The listing builds one solid part. Answer for the finished solid, in the listing's coordinates (mm). Face numbers are marked on the shaded views. A direction names the side the tool comes from. Round coordinates to 2 decimals unless told otherwise and drop trailing zeros. Write each loop counter-clockwise with the first axis right and the second up, starting at its lowest first coordinate (ties: lowest second). Pieces come first, ordered by that corner, then holes. Notation, with made-up numbers: (-38, 2.25) - (8, 2.25) arc R16 cw to (8, 18.25) - close; hole circle Ø7 at (55, 77). An arc over 180 degrees is marked (long way). Return JSON: item names as keys, results as strings. Group by question number.
(1) Which of the six approach directions +Z, -Z, +X, -X, +Y, -Y give full straight-line access (tool end or side, diameter ignored) to the marked faces 1 and 2?
(2) Section D-D, the plane z = 16.5 is taken. Write down the section's boundary in (x, y), then the cut area to 3 significant figures.
(3) Section C-C, the plane x = 2.25 is taken. Write down the section's boundary in (y, z), then the cut area to 3 significant figures.
(4) Determine the mould class of the marked faces 3, 4, 5 and 6 for opening direction Z: +Z half, -Z half, draft (parallel to the pull), parting line (faces both ways), or undercut.
(5) Each of these flat-tipped pins is pushed along its axis until it touches: pin 1 (8.5 mm diameter, centred on y = 11, z = 10, fed in from -X); pin 2 (3.5 mm diameter, centred on x = 6, z = 6, fed in from -Y). Where does it stop, or does it pass through?
(6) Find the intervals of material crossed by line 1 along Y through (x, z) = (1.8, 14.75); line 2 along Y through (x, z) = (4.75, 10); line 3 along X through (y, z) = (6.5, 10.5), in increasing order. Write a range as [from, to].
(7) Section A-A, the plane y = 11 is taken. Write down the section's boundary in (x, z), then the cut area to 3 significant figures.
(8) Section B-B, the plane z = 10 is taken. Write down the section's boundary in (x, y).
```python
from build123d import *

# Parameters (mm, degrees)
BOSS_EXTRUDE1_DEPTH = 20
CUT_EXTRUDE1_REACH  = 9
SKETCH2_R           = 2.6
CUT_EXTRUDE2_REACH  = 6
SKETCH3_R           = 1.25


with BuildPart() as part:
    # Sketch1 → Boss-Extrude1 (new body)
    with BuildSketch(Plane.XY):
        Polygon((7, 15), (0, 15), (0, 0), (4, 0), (4, 7), (7, 7), align=None)
    extrude(amount=BOSS_EXTRUDE1_DEPTH)

    # Sketch2 → Cut-Extrude1 (cut, up to next)
    with BuildSketch(Plane(origin=(7, 0, 0), x_dir=(0, 0, -1), z_dir=(1, 0, 0)), mode=Mode.PRIVATE) as cut_extrude1_sk1:
        with Locations((-10, 11)):
            Circle(SKETCH2_R)
    cut_extrude1_tool1 = extrude(cut_extrude1_sk1.sketch, amount=-CUT_EXTRUDE1_REACH, mode=Mode.PRIVATE) & part.part
    add(cut_extrude1_tool1.solids().sort_by_distance((7, 11, 10))[0], mode=Mode.SUBTRACT)

    # Sketch3 → Cut-Extrude2 (cut, up to next)
    with BuildSketch(Plane(origin=(4, 0, 0), x_dir=(0, 0, -1), z_dir=(1, 0, 0)), mode=Mode.PRIVATE) as cut_extrude2_sk1:
        with Locations((-14.75, 3.497875885)):
            Circle(SKETCH3_R)
    cut_extrude2_tool1 = extrude(cut_extrude2_sk1.sketch, amount=-CUT_EXTRUDE2_REACH, mode=Mode.PRIVATE) & part.part
    add(cut_extrude2_tool1.solids().sort_by_distance((4, 3.497876, 14.75))[0], mode=Mode.SUBTRACT)
    # Sketch3 → Cut-Extrude2 (cut, up to next)
    with BuildSketch(Plane(origin=(4, 0, 0), x_dir=(0, 0, -1), z_dir=(1, 0, 0)), mode=Mode.PRIVATE) as cut_extrude2_sk2:
        with Locations((-5.25, 3.497875885)):
            Circle(SKETCH3_R)
    cut_extrude2_tool2 = extrude(cut_extrude2_sk2.sketch, amount=-CUT_EXTRUDE2_REACH, mode=Mode.PRIVATE) & part.part
    add(cut_extrude2_tool2.solids().sort_by_distance((4, 3.497876, 5.25))[0], mode=Mode.SUBTRACT)


solid = part.part
```
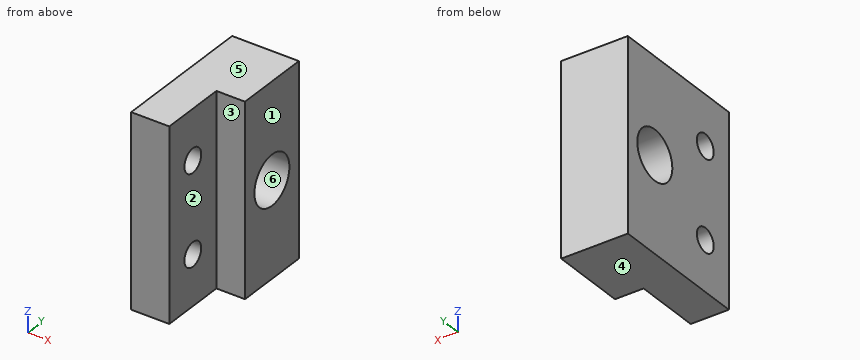
Working result:
{
 "1": {"face 1": "+Z, -Z, +X, +Y, -Y", "face 2": "+Z, -Z, +X, -Y"},
 "2": {"outline": "(0, 0) - (4, 0) - (4, 7) - (7, 7) - (7, 15) - (0, 15) - close", "area": "84.0 mm^2"},
 "3": {"outline": "(0, 0) - (15, 0) - (15, 20) - (0, 20) - close; hole circle Ø2.5 at (3.5, 5.25); hole circle Ø2.5 at (3.5, 14.75); hole circle Ø5.2 at (11, 10)", "area": "269 mm^2"},
 "4": {"face 3": "draft", "face 4": "-Z half", "face 5": "+Z half", "face 6": "undercut"},
 "5": {"pin 1": "stops at x = 0", "pin 2": "stops at y = 7"},
 "6": {"line 1": "y = [0, 2.25], [4.75, 15]", "line 2": "y = [7, 8.4], [13.6, 15]", "line 3": "x = [0, 4]"},
 "7": {"outline": "(0, 0) - (7, 0) - (7, 7.4) - (0, 7.4) - close; (0, 12.6) - (7, 12.6) - (7, 20) - (0, 20) - close", "area": "104 mm^2"},
 "8": {"outline": "(0, 0) - (4, 0) - (4, 7) - (7, 7) - (7, 8.4) - (0, 8.4) - close; (0, 13.6) - (7, 13.6) - (7, 15) - (0, 15) - close"}
}
